Design review of the part built by this model. Coordinates are the model's own, in mm. Coordinates: 2 decimals unless noted, no trailing zeros. Write each loop counter-clockwise with the first axis right and the second up, starting at its lowest first coordinate (ties: lowest second). Pieces come first, ordered by that corner, then holes. Notation, with made-up numbers: (-12, 9) -> (8, 9) arc R31 cw to (8, 43) -> close; hole circle Ø1 at (79.25, 36.25). An arc over 180 degrees is marked (long way). Answer in a Markdown table with one row per item. Add a question column.
Item 1: Take a section at D-D, the plane z = 4. Write out the cut boundary in (x, y), and give its area (3 significant figures).
Item 2: Draft analysis for pull direction Y (two halves, no side actions). For faces 1 (the face through (-0.867, -3.905, 3.088)), 2 (the face through (6.098, -1.858, 3.081)), 3 (the face through (4.66, 4.35, 3.08)), 4 (the face through (0, -5, 6.25)), state which applies: released by +Y, released by -Y, zero draft, split by the parting line, or undercut.
Item 3: To check wall thickness, follow line 1 (Y direction, x = 0, z = 3.55); line 2 (X direction, y = -2, z = 6); line 3 (X direction, y = 2, z = 1.5). State the ranges of each line that lie inside material, in increasing order.
Item 4: Take a section at A-A, the plane z = 6. Write out the cut boundary in (x, y), and give its area (3 significant figures).
Item 5: Take a section at B-B, the plane y = 0. Write out the cut boundary in (x, z), and give its area (3 significant figures).
Item 6: Take a section at C-C, the plane x = 0. Write out the cut boundary in (y, z).
Item 7: Clearance check with a flat-ended pin moving along its axis: P1, Ø1.5, axis at x = 5.5, y = -2, coming from the -Z side. State where the tip first meets the part, or that it passes through.
from build123d import *

# Parameters (mm, degrees)
SKETCH1_R       = 4
NUT_DEPTH       = 6.25
CHANFREIN1_SIZE = 0.5


with BuildPart() as part:
    # Sketch1 → NUT (new body)
    with BuildSketch(Plane.XY):
        Polygon((-5.068605871, 5.338233277), (-7.157348565, -1.720424807), (-2.088742694, -7.058658085), (5.068605871, -5.338233277), (7.157348565, 1.720424807), (2.088742694, 7.058658085), align=None)
        Circle(SKETCH1_R, mode=Mode.SUBTRACT)
    extrude(amount=NUT_DEPTH)

    # Chanfrein1
    chanfrein1_edges = [part.edges().sort_by_distance(p)[0] for p in [
        (-4, 0, 0),
        (-4, 0, 6.25),
    ]]
    chamfer(chanfrein1_edges, length=CHANFREIN1_SIZE)


solid = part.part
Answers:
| question | item | result |
|---|---|---|
| 1 | outline | (-7.16, -1.72) -> (-2.09, -7.06) -> (5.07, -5.34) -> (7.16, 1.72) -> (2.09, 7.06) -> (-5.07, 5.34) -> close; hole circle Ø8 at (0, 0) |
| 1 | area | 90.5 mm^2 |
| 2 | face 1 | undercut |
| 2 | face 2 | released by -Y |
| 2 | face 3 | released by +Y |
| 2 | face 4 | zero draft |
| 3 | line 1 | y = -6.56 to -4, 4 to 6.56 |
| 3 | line 2 | x = -6.89 to -3.75, 3.75 to 6.06 |
| 3 | line 3 | x = -6.06 to -3.46, 3.46 to 6.89 |
| 4 | outline | (-7.16, -1.72) -> (-2.09, -7.06) -> (5.07, -5.34) -> (7.16, 1.72) -> (2.09, 7.06) -> (-5.07, 5.34) -> close; hole circle Ø8.5 at (0, 0) |
| 4 | area | 84.0 mm^2 |
| 5 | outline | (-6.65, 0) -> (-4.5, 0) -> (-4, 0.5) -> (-4, 5.75) -> (-4.5, 6.25) -> (-6.65, 6.25) -> close; (4, 0.5) -> (4.5, 0) -> (6.65, 0) -> (6.65, 6.25) -> (4.5, 6.25) -> (4, 5.75) -> close |
| 5 | area | 32.6 mm^2 |
| 6 | outline | (-6.56, 0) -> (-4.5, 0) -> (-4, 0.5) -> (-4, 5.75) -> (-4.5, 6.25) -> (-6.56, 6.25) -> close; (4, 0.5) -> (4.5, 0) -> (6.56, 0) -> (6.56, 6.25) -> (4.5, 6.25) -> (4, 5.75) -> close |
| 7 | P1 | stops at z = 0 |
